Read the model definition and answer for the solid it produces. Units are mm, in the model's axes. A direction names the side the tool comes from. Give positions to 0.01 mm unless a question says otherwise; leave off trailing zeros. Order: outer loops, then holes, each group sorted by start corner. A loop starts at its lowest first (then second) coordinate and runs counter-clockwise, first axis right, second up. Notation, with made-up numbers: (89.25, -38.75) -> (112.25, -38.75) arc R28 ccw to (112.25, -12.75) -> close; hole circle Ø1 at (11.5, 86). An arc over 180 degrees is marked (long way). Use one line per item in the form item = value.
```python
from build123d import *

# Parameters (mm, degrees)
EXTRUDE_1_DEPTH     = 2
EXTRUDE_START       = -2
SKETCH_2_W          = 14
SKETCH_2_H          = 13
SKETCH_2_R          = 1.5
EXTRUDE_2_DEPTH     = 4.5
SKETCH_3_W          = 1.5
SKETCH_3_H          = 1.268219588
EXTRUDE_3_DEPTH     = 13
SKETCH_4_W          = 1.5
SKETCH_4_H          = 1
EXTRUDE_4_DEPTH     = 11.463560824
CUT_EXTRUDE_1_REACH = 39.756
SKETCH_5_W          = 1.5
SKETCH_5_H          = 14
SKETCH_7_W          = 4
SKETCH_7_H          = 1
EXTRUDE_5_DEPTH     = 13
CUT_EXTRUDE_START   = 0.5
SKETCH_6_R          = 5
CUT_EXTRUDE_2_DEPTH = 4
CUT_EXTRUDE_3_DEPTH = 49


with BuildPart() as part:
    # Эскиз1 → Бобышка-Вытянуть1 (new body)
    with BuildSketch(Plane(origin=(0, 0, 0), x_dir=(1, 0, 0), z_dir=(0, 1, 0))):
        Polygon((16, -4.5), (16, -24.5), (-16, -24.5), (-16, -4.5), (-24.5, -4.5), (-24.5, 24.5), (24.5, 24.5), (24.5, -4.5), align=None)
    extrude(amount=EXTRUDE_1_DEPTH)

    # Эскиз2 → Бобышка-Вытянуть2 (add)
    with BuildSketch(Plane(origin=(16, 0, 0), x_dir=(0, 0, -1), z_dir=(1, 0, 0)).offset(EXTRUDE_START)):
        with Locations((-17.5, 8.5)):
            Rectangle(SKETCH_2_W, SKETCH_2_H)
        with Locations((-15.5, 8)):
            Circle(SKETCH_2_R, mode=Mode.SUBTRACT)
    extrude(amount=-EXTRUDE_2_DEPTH)

    # Эскиз3 → Бобышка-Вытянуть3 (add)
    with BuildSketch(Plane(origin=(0, 15, 0), x_dir=(1, 0, 0), z_dir=(0, 1, 0))):
        with Locations((8.75, -11.134109794)):
            Rectangle(SKETCH_3_W, SKETCH_3_H)
        with Locations((8.75, -23.865890206)):
            Rectangle(SKETCH_3_W, SKETCH_3_H)
    extrude(amount=-EXTRUDE_3_DEPTH)

    # Эскиз4 → Бобышка-Вытянуть4 (add)
    with BuildSketch(Plane.XY.offset(11.768219588)):
        with Locations((8.75, 2.5)):
            Rectangle(SKETCH_4_W, SKETCH_4_H)
    extrude(amount=EXTRUDE_4_DEPTH)

    # Вырез-Вытянуть1: up to this face of the body (flat: up to its plane)
    cut_extrude_1_end = Plane(part.part.faces().sort_by_distance((-0.46737481, 2, -3.237228123))[0])
    # Эскиз5 → Вырез-Вытянуть1 (cut, up to the picked face)
    with BuildSketch(Plane(origin=(0, 15, 0), x_dir=(1, 0, 0), z_dir=(0, 1, 0)), mode=Mode.PRIVATE) as cut_extrude_1_sk1:
        with Locations((13.25, -17.5)):
            Rectangle(SKETCH_5_W, SKETCH_5_H)
    cut_extrude_1_tool1 = split(extrude(cut_extrude_1_sk1.sketch, amount=-CUT_EXTRUDE_1_REACH, mode=Mode.PRIVATE), bisect_by=cut_extrude_1_end, keep=Keep.BOTH, mode=Mode.PRIVATE)
    add(cut_extrude_1_tool1.solids().sort_by(Axis((13.25, 15, 17.5), (0, -1, 0)))[0], mode=Mode.SUBTRACT)

    # Эскиз7 → Бобышка-Вытянуть5 (add)
    with BuildSketch(Plane(origin=(0, 15, 0), x_dir=(1, 0, 0), z_dir=(0, 1, 0))):
        with Locations((10.5, -10)):
            Rectangle(SKETCH_7_W, SKETCH_7_H)
    extrude(amount=-EXTRUDE_5_DEPTH)

    # Эскиз6 → Вырез-Вытянуть2 (cut)
    with BuildSketch(Plane(origin=(12.5, 0, 0), x_dir=(0, 0, -1), z_dir=(1, 0, 0)).offset(CUT_EXTRUDE_START)):
        with Locations(Location((-15.5, 8, 0), (0, 0, 270))):
            Circle(SKETCH_6_R)
    extrude(amount=-CUT_EXTRUDE_2_DEPTH, mode=Mode.SUBTRACT)

    # Эскиз8 → Вырез-Вытянуть3 (cut)
    with BuildSketch(Plane(origin=(24.5, 0, 0), x_dir=(0, 0, -1), z_dir=(1, 0, 0))):
        Polygon((24.5, 0), (22.5, 2), (24.5, 2), align=None)
    extrude(amount=-CUT_EXTRUDE_3_DEPTH, mode=Mode.SUBTRACT)


solid = part.part
```
Item 1: Determine the mould class of faces 1 (the flat face through (9, 8, 11)), 2 (the flat face through (16, 1, 14)), 3 (the flat face through (0.3, 1, -23.5)) for opening direction Z: +Z half, -Z half, draft (parallel to the pull), parting line (faces both ways), or undercut.
Checks:
face_1 = undercut
face_2 = draft
face_3 = -Z half
Item 2: Straight lines are drawn through the part: L1, parallel to Z at x = 10.9, y = 8; L2, parallel to Y at x = 7.5, z = -0.5; L3, parallel to Z at x = 11.5, y = 11. For each, find the intervals that lie inside material, in ascending order. Write a range as from..to.
Checks:
L1 = 9.5..10.5, 20.5..24.5
L2 = 0..2
L3 = 9.5..11.5, 19.5..24.5
Item 3: The part is cut by section D-D on z = -11. Give the vertices of the cut face in (x, y).
Checks:
outline = (-24.5, 0) -> (24.5, 0) -> (24.5, 2) -> (-24.5, 2) -> close
Item 4: The part is cut by section B-B on y = 4. Give the vertices of the cut face in (x, z).
Checks:
outline = (8, 10.5) -> (8.5, 10.5) -> (8.5, 9.5) -> (12.5, 9.5) -> (12.5, 12.5) -> (9.5, 12.5) -> (9.5, 11.77) -> (8, 11.77) -> close; (8, 23.23) -> (9.5, 23.23) -> (9.5, 18.5) -> (12.5, 18.5) -> (12.5, 24.5) -> (8, 24.5) -> close
Item 5: The part is cut by section A-A on y = 8. Give the vertices of the cut face in (x, z), and give its area (3 significant figures).
Checks:
outline = (8, 10.5) -> (8.5, 10.5) -> (8.5, 9.5) -> (12.5, 9.5) -> (12.5, 10.5) -> (9, 10.5) -> (9, 11.77) -> (8, 11.77) -> close; (8, 23.23) -> (9.5, 23.23) -> (9.5, 20.5) -> (12.5, 20.5) -> (12.5, 24.5) -> (8, 24.5) -> close
area = 19.2 mm²
Item 6: The part is cut by section C-C on x = -7. Give the vertices of the cut face in (y, z).
Checks:
outline = (0, -24.5) -> (2, -22.5) -> (2, 24.5) -> (0, 24.5) -> close
Item 7: Which of the six approach directions +Z, -Z, +X, -X, +Y, -Y give full straight-line access (tool end or side, diameter ignored) to faces 4 (the flat face through (20, 1, 4.5)), 5 (the flat face through (12.5, 10, 20.4)), 6 (the flat face through (8.6, 9.1, 11.768)), 7 (the flat face through (-16, 1, 15)), 8 (the flat face through (10, 9, 9.5))?
Checks:
face_4 = +Z, +X, +Y, -Y
face_5 = +Z, -Z, +X, +Y
face_6 = -X, +Y
face_7 = +Z, -X, +Y, -Y
face_8 = -Z, +X, -X, +Y
Item 8: Given pin 1 Ø8 at (y, z) = (6.5, 3.5) entering from -X; pin 2 Ø0.6 at (x, y) = (20, 0.5) entering from +Z; pin 3 Ø6 at (y, z) = (10.5, 16.5) entering from -X; pin 4 Ø1 at (y, z) = (1, 18) entering from -X, each flat-ended and moving along its own axis, determine where each tip first touches the part or whether it passes through.
Checks:
pin_1 = through
pin_2 = 4.5
pin_3 = 9.5
pin_4 = -16
